Part print with two shaded views. Sizes in mm from the minimum x, y, z corner. Give positions to 0.01 mm unless a question says otherwise; leave off trailing zeros. Write each loop counter-clockwise with the first axis right and the second up, starting at its lowest first coordinate (ties: lowest second). Pieces come first, ordered by that corner, then holes.
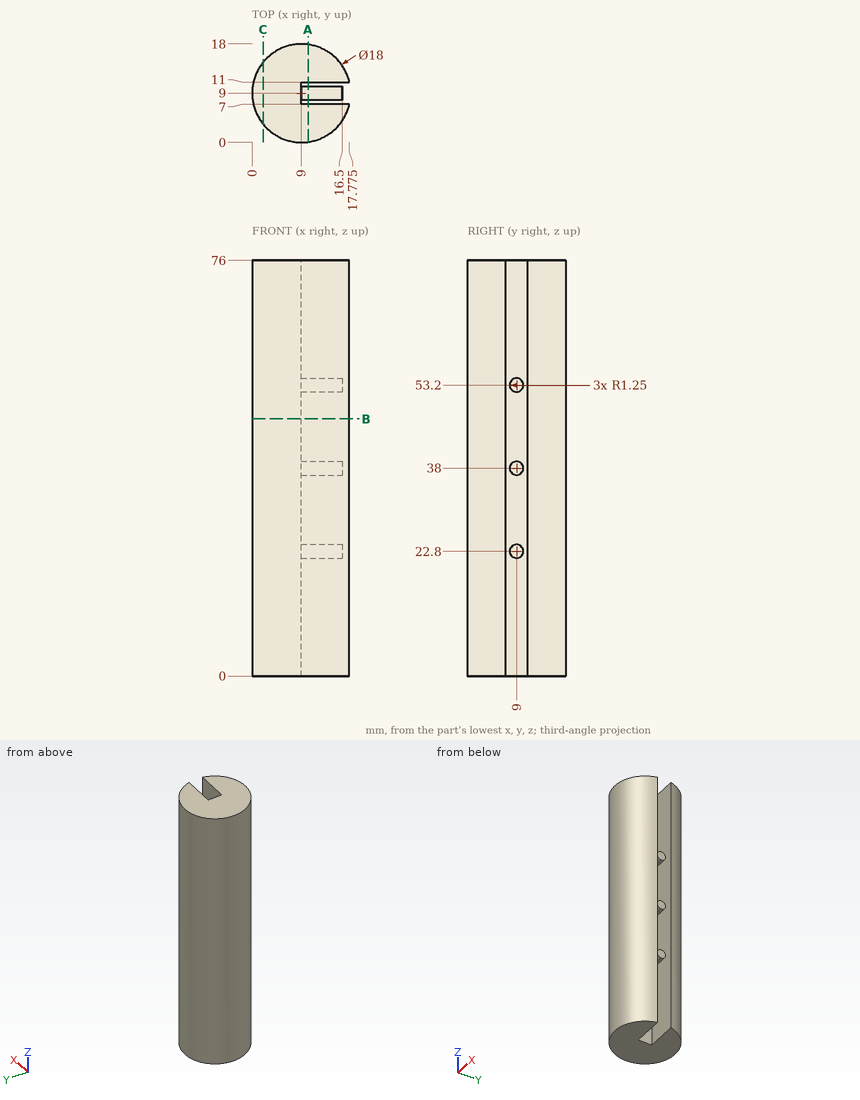
1) Flat gauge pins, fed straight in: P1, Ø1.2, axis at y = 10, z = 47, coming from the +X side; P2, Ø2.5, axis at x = 12.5, z = 54.5, coming from the -Y side; P3, Ø1.2, axis at y = 9.5, z = 53, coming from the +X side. Where does each tip first touch, or does it go through?
Check result:
P1: stops at x = 9
P2: stops at y = 0.29
P3: stops at x = 16.5
2) Saw through at A-A (x = 10.25). Write the cut outline in (y, z).
Check result:
outline: (0.09, 0) - (7, 0) - (7, 76) - (0.09, 76) - close; (9, 21.55) arc R1.25 ccw to (10.25, 22.8) arc R1.25 ccw to (9, 24.05) arc R1.25 ccw to start; (9, 36.75) arc R1.25 ccw to (10.25, 38) arc R1.25 ccw to (9, 39.25) arc R1.25 ccw to start; (9, 51.95) arc R1.25 ccw to (10.25, 53.2) arc R1.25 ccw to (9, 54.45) arc R1.25 ccw to start; (11, 0) - (17.91, 0) - (17.91, 76) - (11, 76) - close
3) Saw through at C-C (x = 2). Write the cut outline in (y, z).
Check result:
outline: (3.34, 0) - (14.66, 0) - (14.66, 76) - (3.34, 76) - close
4) Saw through at B-B (z = 47). Write the cut outline in (x, y) (3 decimals), and give its area (3 significant figures).
Check result:
outline: (9, 7) - (9, 11) - (17.775, 11) arc R9 ccw (long way) to (17.775, 7) - close
area: 219 mm2
5) Drill centre lines: L1, parallel to Y at x = 14.5, z = 38.5; L2, parallel to Z at x = 14, y = 9.25; L3, parallel to Y at x = 11.25, z = 65. Where is each one in solid material? Low to high.
Check result:
L1: y = 1.88 to 7, 7.85 to 10.15, 11 to 16.12
L2: z = 21.58 to 24.02, 36.78 to 39.22, 51.98 to 54.42
L3: y = 0.29 to 7, 11 to 17.71
